Geometry: final body of the model. Coordinates: model frame, mm. A direction names the side the tool comes from. Give positions to 0.01 mm unless a question says otherwise; leave off trailing zeros. Write each loop counter-clockwise with the first axis right and the second up, starting at its lowest first coordinate (ties: lowest second). Pieces come first, ordered by that corner, then holes. Notation, with made-up numbers: M 4,-4.75 L 19,-4.75 A12 ccw 19,0.25 Z; hole C -23.75,-22.5 d8. An arc over 180 degrees is marked long. Answer as a JSON object with one key per item and string values.
from build123d import *

# Parameters (mm, degrees)
SKETCH1_W           = 35
SKETCH1_H           = 19.5
BOSS_EXTRUDE1_DEPTH = 6.45
SKETCH2_W           = 13
SKETCH2_H           = 44
BOSS_EXTRUDE2_DEPTH = 18
SKETCH3_R           = 3.5
CUT_EXTRUDE1_DEPTH  = 19
SKETCH4_W           = 25
SKETCH4_H           = 6
BOSS_EXTRUDE3_DEPTH = 2.6
SKETCH5_R           = 1.4
CUT_EXTRUDE2_DEPTH  = 10.05


with BuildPart() as part:
    # Sketch1 → Boss-Extrude1 (new body)
    with BuildSketch(Plane(origin=(0, 0, 0), x_dir=(1, 0, 0), z_dir=(0, 1, 0))):
        Rectangle(SKETCH1_W, SKETCH1_H)
    extrude(amount=BOSS_EXTRUDE1_DEPTH)

    # Sketch2 → Boss-Extrude2 (add)
    with BuildSketch(Plane(origin=(0, 0, 0), x_dir=(1, 0, 0), z_dir=(0, 1, 0))):
        with Locations((-1, 30.75)):
            Rectangle(SKETCH2_W, SKETCH2_H)
    extrude(amount=BOSS_EXTRUDE2_DEPTH)

    # Sketch3 → Cut-Extrude1 (cut, through all)
    with BuildSketch(Plane(origin=(0, 18, 0), x_dir=(1, 0, 0), z_dir=(0, 1, 0))):
        with Locations((-1, 45.25)):
            Circle(SKETCH3_R)
        with Locations((-1, 15.25)):
            Circle(SKETCH3_R)
    extrude(amount=-CUT_EXTRUDE1_DEPTH, mode=Mode.SUBTRACT)

    # Sketch4 → Boss-Extrude3 (add)
    with BuildSketch(Plane(origin=(0, 6.45, 0), x_dir=(1, 0, 0), z_dir=(0, 1, 0))):
        with Locations((-5, -6.75)):
            Rectangle(SKETCH4_W, SKETCH4_H)
    extrude(amount=BOSS_EXTRUDE3_DEPTH)

    # Sketch5 → Cut-Extrude2 (cut, through all)
    with BuildSketch(Plane(origin=(0, 9.05, 0), x_dir=(1, 0, 0), z_dir=(0, 1, 0))):
        with Locations((-14.5, -6.75)):
            Circle(SKETCH5_R)
        with Locations((4.5, -6.75)):
            Circle(SKETCH5_R)
    extrude(amount=-CUT_EXTRUDE2_DEPTH, mode=Mode.SUBTRACT)


solid = part.part
1) Pull-direction query (Z, two-part tool) for faces 4 (the flat face through (5.5, 9, -30)), 5 (the cylindrical face through (-1.46, 9.13, -48.72)), 6 (the flat face through (-1, 9, -52.75)); classes: pulls with the +Z half, pulls with the -Z half, needs draft (parallel to the pull), parting line crosses it, or undercut.
Geometry check:
{"face 4": "needs draft", "face 5": "undercut", "face 6": "pulls with the -Z half"}
2) Line query: line 1 (X direction, y = 13.5, z = -15.25); line 2 (Z direction, x = -14.5, y = 4.5); line 3 (Z direction, x = 3, y = 7.75). Output: solid intervals per line, ascending. Write a range as from..to.
Geometry check:
{"line 1": "x = -7.5..-4.5, 2.5..5.5", "line 2": "z = -9.75..5.35, 8.15..9.75", "line 3": "z = -52.75..-8.75, 3.75..9.75"}
3) Cut plane B-B on y = 7.25. Return loops of the section in (x, z).
Geometry check:
{"outline": "M -17.5,3.75 L 7.5,3.75 L 7.5,9.75 L -17.5,9.75 Z; M -7.5,-52.75 L 5.5,-52.75 L 5.5,-8.75 L -7.5,-8.75 Z; hole C -14.5,6.75 d2.8; hole C -1,-45.25 d7; hole C -1,-15.25 d7; hole C 4.5,6.75 d2.8"}
4) Set-up query: faces 1 (the flat face through (-1, 12, -8.75)), 2 (the flat face through (-13, 3, -9.75)), 3 (the flat face through (7.5, 8, 7)). Return all of +Z, -Z, +X, -X, +Y, -Y with unobstructed straight access to the full face (end or side cutting, diameter ignored); none if empty.
Geometry check:
{"face 1": "+X, -X, +Y", "face 2": "-Z, -X, +Y, -Y", "face 3": "+Z, -Z, +X, +Y"}
5) Cut plane C-C on z = 6.75. Return loops of the section in (x, y), and give its area (3 significant figures).
Geometry check:
{"outline": "M -17.5,0 L -15.9,0 L -15.9,9.05 L -17.5,9.05 Z; M -13.1,0 L 3.1,0 L 3.1,9.05 L -13.1,9.05 Z; M 5.9,0 L 17.5,0 L 17.5,6.45 L 7.5,6.45 L 7.5,9.05 L 5.9,9.05 Z", "area": "240 mm2"}
6) Cut plane A-A on x = -14.5. Return loops of the section in (y, z).
Geometry check:
{"outline": "M 0,-9.75 L 6.45,-9.75 L 6.45,3.75 L 9.05,3.75 L 9.05,5.35 L 0,5.35 Z; M 0,8.15 L 9.05,8.15 L 9.05,9.75 L 0,9.75 Z"}
7) Cut plane D-D on z = -15.25. Return loops of the section in (x, y).
Geometry check:
{"outline": "M -7.5,0 L -4.5,0 L -4.5,18 L -7.5,18 Z; M 2.5,0 L 5.5,0 L 5.5,18 L 2.5,18 Z"}
8) Contact query for flat-ended pins moving along their axis: P1, Ø1.5, axis at y = 11.5, z = -36.5, coming from the -X side; P2, Ø5.5, axis at y = 8.5, z = -39, coming from the +X side; P3, Ø5, axis at x = -11, y = 4.5, coming from the -Z side. Output: stop coordinate, or through.
Geometry check:
{"P1": "stops at x = -7.5", "P2": "stops at x = 5.5", "P3": "stops at z = -9.75"}
